Work out the finished part from the listing and answer in its coordinate system (mm). A direction names the side the tool comes from. Give positions to 0.01 mm unless a question says otherwise; leave off trailing zeros. Order: outer loops, then holes, each group sorted by start corner. A loop starts at its lowest first (then second) coordinate and runs counter-clockwise, first axis right, second up.
```python
from build123d import *
from build123d.topology import SkipClean

# Parameters (mm, degrees)
SKETCH1_R               = 4
SKETCH1_R_2             = 2
BOSS_EXTRUDE2_DEPTH     = 6.038447986
BOSS_EXTRUDE2_2_DEPTH   = 6.038447986
BOSS_EXTRUDE2_3_DEPTH   = 6.038447986
BOSS_EXTRUDE2_4_DEPTH   = 6.038447986
SKETCH3_W               = 74
SKETCH3_H               = 51.7
BOSS_EXTRUDE4_DEPTH     = 3
BOSS_EXTRUDE3_START     = 11.7
SKETCH2_W               = 8
SKETCH2_H               = 8
SKETCH2_R               = 2
SKETCH2_H_2             = 14
BOSS_EXTRUDE3_DEPTH     = 5
SKETCH1_4_R             = 2
SKETCH1_4_R_2           = 13
CUT_EXTRUDE1_DEPTH      = 10
BOSS_EXTRUDE5_DEPTH     = 8
BOSS_EXTRUDE7_DEPTH     = 8
SKETCH2_2_R             = 2
CUT_EXTRUDE2_DEPTH      = 85.324276113
CUT_EXTRUDE3_START      = -6
SKETCH5_R               = 3.5
SKETCH5_R_2             = 3
CUT_EXTRUDE3_DEPTH      = 72.702596752
BOSS_EXTRUDE8_START     = -4
SKETCH3_3_W             = 58
SKETCH3_3_H             = 35
SKETCH3_3_R             = 4
SKETCH3_3_W_2           = 74
SKETCH3_3_H_2           = 5
BOSS_EXTRUDE8_DEPTH     = 4
CUT_EXTRUDE5_DEPTH      = 79.663462115
CUT_EXTRUDE5_DEPTH_BACK = 79.663462115
SKETCH1_6_R             = 13
SKETCH8_W               = 8
SKETCH8_H               = 14
SKETCH8_H_2             = 11.313736344
CUT_EXTRUDE6_DEPTH      = 25
BOSS_EXTRUDE10_START    = -8
SKETCH9_W               = 10
SKETCH9_H               = 5
BOSS_EXTRUDE10_DEPTH    = 8
SKETCH2_3_R             = 2
CUT_EXTRUDE7_DEPTH      = 25
SKETCH10_R              = 2
CUT_EXTRUDE8_DEPTH      = 25
SKETCH2_4_R             = 2
CUT_EXTRUDE9_DEPTH      = 25
SKETCH1_7_R             = 2
CUT_EXTRUDE10_DEPTH     = 25


with BuildPart() as part:
    # Sketch1 → Boss-Extrude2 (new body)
    with BuildSketch(Plane.XY):
        with Locations((49, 35.83595021)):
            Circle(SKETCH1_R)
        with Locations((49, 35.83595021)):
            Circle(SKETCH1_R_2, mode=Mode.SUBTRACT)
    extrude(amount=BOSS_EXTRUDE2_DEPTH)



with BuildPart() as body_2:
    # Sketch1 → Boss-Extrude2 2 (new body)
    with BuildSketch(Plane.XY):
        with Locations((49, 7.83595021)):
            Circle(SKETCH1_R)
        with Locations((49, 7.83595021)):
            Circle(SKETCH1_R_2, mode=Mode.SUBTRACT)
    extrude(amount=BOSS_EXTRUDE2_2_DEPTH)


with BuildPart() as body_3:
    # Sketch1 → Boss-Extrude2 3 (new body)
    with BuildSketch(Plane.XY):
        with Locations((9, 7.83595021)):
            Circle(SKETCH1_R)
        with Locations((9, 7.83595021)):
            Circle(SKETCH1_R_2, mode=Mode.SUBTRACT)
    extrude(amount=BOSS_EXTRUDE2_3_DEPTH)


with BuildPart() as body_4:
    # Sketch1 → Boss-Extrude2 4 (new body)
    with BuildSketch(Plane.XY):
        with Locations((9, 35.83595021)):
            Circle(SKETCH1_R)
        with Locations((9, 35.83595021)):
            Circle(SKETCH1_R_2, mode=Mode.SUBTRACT)
    extrude(amount=BOSS_EXTRUDE2_4_DEPTH)


with BuildPart() as part_1:
    add(part.part)

    add(body_2.part)  # Boss-Extrude4 merges body 2

    add(body_3.part)  # Boss-Extrude4 merges body 3

    add(body_4.part)  # Boss-Extrude4 merges body 4
    # Sketch3 → Boss-Extrude4 (add)
    with BuildSketch(Plane.XY.offset(6.038447986)):
        with Locations((29, 15.98595021)):
            Rectangle(SKETCH3_W, SKETCH3_H)
    extrude(amount=BOSS_EXTRUDE4_DEPTH)

    # Sketch2 → Boss-Extrude3 (add)
    # profile 1 of 2: a face of its own
    with BuildSketch(Plane(origin=(0, -9.86404979, 0), x_dir=(1, 0, 0), z_dir=(0, 1, 0)).offset(BOSS_EXTRUDE3_START)):
        with Locations((-4, -2.038447986)):
            Rectangle(SKETCH2_W, SKETCH2_H)
        with Locations(Location((-4, -1.038447986, 0), (0, 0, 270))):
            Circle(SKETCH2_R, mode=Mode.SUBTRACT)
    # profile 2 of 2: a face of its own
    with BuildSketch(Plane(origin=(0, -9.86404979, 0), x_dir=(1, 0, 0), z_dir=(0, 1, 0)).offset(BOSS_EXTRUDE3_START)):
        with Locations((62, 0.961552014)):
            Rectangle(SKETCH2_W, SKETCH2_H_2)
        with Locations(Location((62, -1.038447986, 0), (0, 0, 270))):
            Circle(SKETCH2_R, mode=Mode.SUBTRACT)
    extrude(amount=BOSS_EXTRUDE3_DEPTH)

    # Sketch1<4> → Cut-Extrude1 (cut)
    with BuildSketch(Plane.XY):
        with Locations((9, 35.83595021)):
            Circle(SKETCH1_4_R)
        with Locations((9, 7.83595021)):
            Circle(SKETCH1_4_R)
        with Locations((49, 35.83595021)):
            Circle(SKETCH1_4_R)
        with Locations((38.5, 21.83595021)):
            Circle(SKETCH1_4_R_2)
        with Locations((49, 7.83595021)):
            Circle(SKETCH1_4_R)
    extrude(amount=CUT_EXTRUDE1_DEPTH, mode=Mode.SUBTRACT)

    # Sketch4 → Boss-Extrude5 (add)
    with BuildSketch(Plane(origin=(66, 0, 0), x_dir=(0, 0, -1), z_dir=(1, 0, 0))):
        Polygon((7.961552014, 6.83595021), (-6.038447986, 41.83595021), (-6.038447986, 6.83595021), align=None)
    extrude(amount=-BOSS_EXTRUDE5_DEPTH)

    # Sketch6 → Boss-Extrude7 (add)
    with BuildSketch(Plane.ZY.offset(8)):
        Polygon((-1.961552014, 6.83595021), (6.038447986, 14.993789145), (6.038447986, 6.83595021), align=None)
    extrude(amount=-BOSS_EXTRUDE7_DEPTH)

    # Sketch2<2> → Cut-Extrude2 (cut, through all)
    with SkipClean():  # the faces are left unmerged after this step: merging them gives an invalid solid
        with BuildSketch(Plane(origin=(0, -9.86404979, 0), x_dir=(1, 0, 0), z_dir=(0, 1, 0))):
            with Locations(Location((62, -1.038447986, 0), (0, 0, 90))):
                Circle(SKETCH2_2_R)
            with Locations(Location((-4, -1.038447986, 0), (0, 0, 90))):
                Circle(SKETCH2_2_R)
        extrude(amount=CUT_EXTRUDE2_DEPTH, mode=Mode.SUBTRACT)
    add(part_1.part.scale(1), mode=Mode.REPLACE)  # the faces are merged on a copy

    # Sketch5 → Cut-Extrude3 (cut, through all)
    with SkipClean():  # the faces are left unmerged after this step: merging them gives an invalid solid
        with BuildSketch(Plane.XZ.offset(-1.83595021).offset(CUT_EXTRUDE3_START)):
            with Locations(Location((62, 1.038447986, 0), (0, 0, 270))):
                Circle(SKETCH5_R)
            with Locations((-4, 1.038447986)):
                Circle(SKETCH5_R_2)
        extrude(amount=-CUT_EXTRUDE3_DEPTH, mode=Mode.SUBTRACT)

    # Sketch3<3> → Boss-Extrude8 (add)
    # profile 1 of 2: a face of its own
    with BuildSketch(Plane.XY.offset(6.038447986).offset(BOSS_EXTRUDE8_START)):
        with Locations((29, 24.33595021)):
            Rectangle(SKETCH3_3_W, SKETCH3_3_H)
        with Locations((49, 35.83595021)):
            Circle(SKETCH3_3_R, mode=Mode.SUBTRACT)
    # profile 2 of 2: a face of its own
    with BuildSketch(Plane.XY.offset(6.038447986).offset(BOSS_EXTRUDE8_START)):
        with Locations((29, 4.33595021)):
            Rectangle(SKETCH3_3_W_2, SKETCH3_3_H_2)
    extrude(amount=BOSS_EXTRUDE8_DEPTH)

    # Sketch1<6> → Cut-Extrude5 (cut, two sides: drawn at the far end of the back side and taken through both)
    with BuildSketch(Plane.XY.offset(-CUT_EXTRUDE5_DEPTH_BACK)):
        with Locations((38.5, 21.83595021)):
            Circle(SKETCH1_6_R)
    extrude(amount=CUT_EXTRUDE5_DEPTH + CUT_EXTRUDE5_DEPTH_BACK, mode=Mode.SUBTRACT)

    # Sketch8 → Cut-Extrude6 (cut)
    with BuildSketch(Plane(origin=(0, 41.83595021, 0), x_dir=(1, 0, 0), z_dir=(0, 1, 0))):
        with Locations((62, 0.961552014)):
            Rectangle(SKETCH8_W, SKETCH8_H)
        with Locations((-4, -0.381579814)):
            Rectangle(SKETCH8_W, SKETCH8_H_2)
    extrude(amount=-CUT_EXTRUDE6_DEPTH, mode=Mode.SUBTRACT)

    # Sketch9 → Boss-Extrude10 (add)
    with BuildSketch(Plane.ZY.offset(8).offset(BOSS_EXTRUDE10_START)):
        with Locations((1.038447986, 4.33595021)):
            Rectangle(SKETCH9_W, SKETCH9_H)
    extrude(amount=BOSS_EXTRUDE10_DEPTH)

    # Sketch2<3> → Cut-Extrude7 (cut)
    with BuildSketch(Plane(origin=(0, -9.86404979, 0), x_dir=(1, 0, 0), z_dir=(0, 1, 0))):
        with Locations(Location((-4, -1.038447986, 0), (0, 0, 90))):
            Circle(SKETCH2_3_R)
    extrude(amount=CUT_EXTRUDE7_DEPTH, mode=Mode.SUBTRACT)

    # Sketch10 → Cut-Extrude8 (cut)
    with BuildSketch(Plane.XY.offset(9.038447986)):
        with Locations((44, -3.96404979)):
            Circle(SKETCH10_R)
        with Locations((14, -3.96404979)):
            Circle(SKETCH10_R)
    extrude(amount=-CUT_EXTRUDE8_DEPTH, mode=Mode.SUBTRACT)

    # Sketch2<4> → Cut-Extrude9 (cut)
    with BuildSketch(Plane(origin=(0, -9.86404979, 0), x_dir=(1, 0, 0), z_dir=(0, 1, 0))):
        with Locations(Location((62, -1.038447986, 0), (0, 0, 90))):
            Circle(SKETCH2_4_R)
    extrude(amount=CUT_EXTRUDE9_DEPTH, mode=Mode.SUBTRACT)

    # Sketch1<7> → Cut-Extrude10 (cut)
    with BuildSketch(Plane.XY):
        with Locations((9, 35.83595021)):
            Circle(SKETCH1_7_R)
        with Locations((9, 7.83595021)):
            Circle(SKETCH1_7_R)
        with Locations((49, 35.83595021)):
            Circle(SKETCH1_7_R)
        with Locations((49, 7.83595021)):
            Circle(SKETCH1_7_R)
    extrude(amount=CUT_EXTRUDE10_DEPTH, mode=Mode.SUBTRACT)


solid = part_1.part
```
1. The part is cut by section A-A (x = 38.5). Write down the section's boundary in (y, z), then the cut area to 3 significant figures.
Findings below:
outline: (-9.86, 6.04) - (1.84, 6.04) - (1.84, 2.04) - (8.84, 2.04) - (8.84, 9.04) - (-9.86, 9.04) - close; (34.84, 2.04) - (41.84, 2.04) - (41.84, 9.04) - (34.84, 9.04) - close
area: 133 mm2
2. Given P1, Ø9, axis at x = -3.5, y = 27, coming from the -Z side; P2, Ø2.5, axis at x = 9.5, y = 6.5, coming from the -Z side; P3, Ø10, axis at x = 45, z = -3.5, coming from the -Y side, each flat-ended and moving along its own axis, determine where each tip first touches the part or whether it passes through.
Findings below:
P1: stops at z = 2.04
P2: stops at z = 0
P3: stops at y = 3.86
3. The mould has two halves that part along Z. Classify faces 6 (the face through (-5.83, 12.67, 3.76)), 7 (the face through (-8, 12, 5)), 8 (the face through (-4, 7.836, 3.2)): pulls with the +Z half, pulls with the -Z half, needs draft (parallel to the pull), parting line crosses it, or undercut.
Findings below:
face 6: pulls with the -Z half
face 7: needs draft
face 8: undercut
4. The part is cut by section D-D (x = 9). Write down the section's boundary in (y, z), then the cut area to 3 significant figures.
Findings below:
outline: (-9.86, 6.04) - (1.84, 6.04) - (1.84, 2.04) - (3.84, 2.04) - (3.84, 0) - (5.84, 0) - (5.84, 9.04) - (-9.86, 9.04) - close; (9.84, 0) - (11.84, 0) - (11.84, 2.04) - (31.84, 2.04) - (31.84, 0) - (33.84, 0) - (33.84, 9.04) - (9.84, 9.04) - close; (37.84, 0) - (39.84, 0) - (39.84, 2.04) - (41.84, 2.04) - (41.84, 9.04) - (37.84, 9.04) - close
area: 275 mm2
5. The part is cut by section B-B (y = 21). Write down the section's boundary in (x, z), then the cut area to 3 significant figures.
Findings below:
outline: (-8, 6.04) - (0, 6.04) - (0, 2.04) - (25.53, 2.04) - (25.53, 9.04) - (-8, 9.04) - close; (51.47, 2.04) - (58, 2.04) - (58, 6.04) - (66, 6.04) - (66, 9.04) - (51.47, 9.04) - close
area: 272 mm2
6. Straight lines are drawn through the part: probe 1 along Y at (x, z) = (9, 8.2); probe 2 along Y at (x, z) = (9, 0.8); probe 3 along Y at (x, z) = (10.5, 3.25). For each, find the intervals that lie inside material, in ascending order.
Findings below:
probe 1: y = -9.86 to 5.84, 9.84 to 33.84, 37.84 to 41.84
probe 2: y = 3.84 to 5.84, 9.84 to 11.84, 31.84 to 33.84, 37.84 to 39.84
probe 3: y = 1.84 to 6.51, 9.16 to 34.51, 37.16 to 41.84
7. The part is cut by section C-C (x = 49). Write down the section's boundary in (y, z).
Findings below:
outline: (-9.86, 6.04) - (1.84, 6.04) - (1.84, 2.04) - (3.84, 2.04) - (3.84, 0) - (5.84, 0) - (5.84, 9.04) - (-9.86, 9.04) - close; (9.84, 0) - (11.84, 0) - (11.84, 2.04) - (14.17, 2.04) - (14.17, 9.04) - (9.84, 9.04) - close; (29.5, 2.04) - (31.84, 2.04) - (31.84, 0) - (33.84, 0) - (33.84, 9.04) - (29.5, 9.04) - close; (37.84, 0) - (39.84, 0) - (39.84, 2.04) - (41.84, 2.04) - (41.84, 9.04) - (37.84, 9.04) - close
8. Which of the six approach directions +Z, -Z, +X, -X, +Y, -Y give full straight-line access (tool end or side, diameter ignored) to faces 1 (the face through (-4, 29, 6.038)), 2 (the face through (28, 11, 9.038)), 3 (the face through (60, 7.836, 0)), 4 (the face through (7, 7, 0)), 5 (the face through (60.2, 16.836, -2.4))?
Findings below:
face 1: -Z, -X, +Y
face 2: +Z, +X, -X, +Y, -Y
face 3: +Y
face 4: -Z, +Y, -Y
face 5: -Z, +X, +Y
